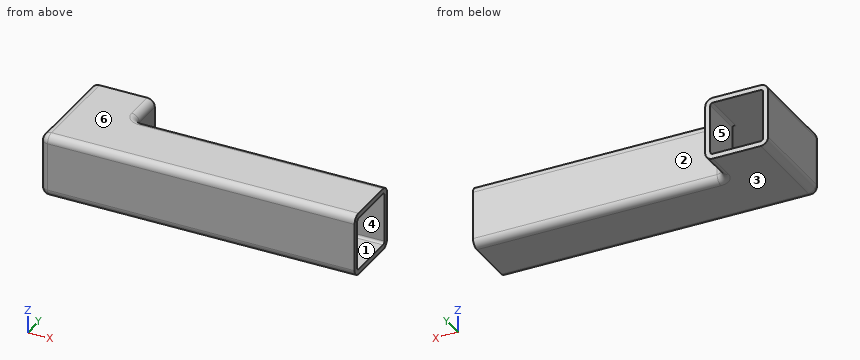
from build123d import *

# Parameters (mm, degrees)
SKETCH1_W           = 125
SKETCH1_H           = 40
BOSS_EXTRUDE1_DEPTH = 25
SKETCH2_W           = 100
SKETCH2_H           = 15
CUT_EXTRUDE1_DEPTH  = 25
SKETCH3_W           = 21
SKETCH3_H           = 21
CUT_EXTRUDE2_DEPTH  = 123
SKETCH4_W           = 21
SKETCH4_H           = 21
CUT_EXTRUDE3_DEPTH  = 38
FILLET3_R           = 1
FILLET4_R           = 1
FILLET5_R           = 1
FILLET6_R           = 1
FILLET7_R           = 1
FILLET8_R           = 1
FILLET9_R           = 3
FILLET11_R          = 3
FILLET12_R          = 3


with BuildPart() as part:
    # Sketch1 → Boss-Extrude1 (new body)
    with BuildSketch(Plane.XY):
        with Locations((62.5, 20)):
            Rectangle(SKETCH1_W, SKETCH1_H)
    extrude(amount=BOSS_EXTRUDE1_DEPTH)

    # Sketch2 → Cut-Extrude1 (cut)
    with BuildSketch(Plane.XY.offset(25)):
        with Locations((75, 32.5)):
            Rectangle(SKETCH2_W, SKETCH2_H)
    extrude(amount=-CUT_EXTRUDE1_DEPTH, mode=Mode.SUBTRACT)

    # Sketch3 → Cut-Extrude2 (cut)
    with BuildSketch(Plane(origin=(125, 0, 0), x_dir=(0, 0, -1), z_dir=(1, 0, 0))):
        with Locations((-12.5, 12.5)):
            Rectangle(SKETCH3_W, SKETCH3_H)
    extrude(amount=-CUT_EXTRUDE2_DEPTH, mode=Mode.SUBTRACT)

    # Sketch4 → Cut-Extrude3 (cut)
    with BuildSketch(Plane(origin=(0, 40, 0), x_dir=(1, 0, 0), z_dir=(0, 1, 0))):
        with Locations((12.5, -12.5)):
            Rectangle(SKETCH4_W, SKETCH4_H)
    extrude(amount=-CUT_EXTRUDE3_DEPTH, mode=Mode.SUBTRACT)

    # Fillet3
    fillet3_edges = [part.edges().sort_by_distance(p)[0] for p in [
        (2, 21, 2),
        (63.5, 2, 2),
    ]]
    fillet(fillet3_edges, radius=FILLET3_R)

    # Fillet4
    fillet4_edges = [part.edges().sort_by_distance(p)[0] for p in [
        (2, 21, 23),
        (63.5, 2, 23),
    ]]
    fillet(fillet4_edges, radius=FILLET4_R)

    # Fillet5
    fillet5_edges = [part.edges().sort_by_distance(p)[0] for p in [
        (74, 23, 2),
    ]]
    fillet(fillet5_edges, radius=FILLET5_R)

    # Fillet6
    fillet6_edges = [part.edges().sort_by_distance(p)[0] for p in [
        (74, 23, 23),
    ]]
    fillet(fillet6_edges, radius=FILLET6_R)

    # Fillet7
    fillet7_edges = [part.edges().sort_by_distance(p)[0] for p in [
        (23, 31, 23),
    ]]
    fillet(fillet7_edges, radius=FILLET7_R)

    # Fillet8
    fillet8_edges = [part.edges().sort_by_distance(p)[0] for p in [
        (23, 31, 2),
    ]]
    fillet(fillet8_edges, radius=FILLET8_R)

    # Fillet9
    fillet9_edges = [part.edges().sort_by_distance(p)[0] for p in [
        (25, 25, 12.5),
        (25, 32.5, 25),
        (75, 25, 25),
        (0, 20, 25),
        (62.5, 0, 25),
    ]]
    fillet(fillet9_edges, radius=FILLET9_R)

    # Fillet11
    fillet11_edges = [part.edges().sort_by_distance(p)[0] for p in [
        (76.5, 25, 0),
        (25.878679656, 25.878679656, 0),
        (25, 34, 0),
        (62.5, 0, 0),
        (0, 20, 0),
    ]]
    fillet(fillet11_edges, radius=FILLET11_R)

    # Fillet12
    # the kernel refuses this fillet: 3 mm, written as the material it takes off along each edge
    with BuildSketch(Plane(origin=(3, 3, 22), x_dir=(-1, 0, 0), z_dir=(0, -1, 0))) as fillet12_piece_1_section:
        Polygon((0, 0), (FILLET12_R, 0), (FILLET12_R, -FILLET12_R), (0, -FILLET12_R), align=None)
    fillet12_piece_1 = extrude(amount=FILLET12_R, mode=Mode.PRIVATE)
    fillet12_piece_1 = fillet12_piece_1 - Plane(origin=(3, 3, 22), x_dir=(0.7071067811865475, 0, -0.7071067811865475), z_dir=(0, -1, 0)) * Sphere(FILLET12_R, mode=Mode.PRIVATE)
    add(fillet12_piece_1, mode=Mode.SUBTRACT)
    with BuildSketch(Plane(origin=(3, 3, 3), x_dir=(-1, 0, 0), z_dir=(0, -1, 0))) as fillet12_piece_2_section:
        Polygon((0, 0), (FILLET12_R, 0), (FILLET12_R, FILLET12_R), (0, FILLET12_R), align=None)
    fillet12_piece_2 = extrude(amount=FILLET12_R, mode=Mode.PRIVATE)
    fillet12_piece_2 = fillet12_piece_2 - Plane(origin=(3, 3, 3), x_dir=(0.7071067811865475, 0, 0.7071067811865475), z_dir=(0, -1, 0)) * Sphere(FILLET12_R, mode=Mode.PRIVATE)
    add(fillet12_piece_2, mode=Mode.SUBTRACT)
    with BuildSketch(Plane(origin=(0, 0, 3), x_dir=(1, 0, 0), z_dir=(0, 0, 1))) as fillet12_piece_3:
        with BuildLine():
            CenterArc((FILLET12_R, FILLET12_R), FILLET12_R, 180, 90)
            Line((0, FILLET12_R), (0, 0))
            Line((0, 0), (FILLET12_R, 0))
        make_face()
    extrude(amount=19, mode=Mode.SUBTRACT)


solid = part.part
Can you work these out from the model? Positions are in its coordinate system, mm. Face numbers are marked on the shaded views. A direction names the side the tool comes from. Give positions to 0.01 mm unless a question says otherwise; leave off trailing zeros. Order: outer loops, then holes, each group sorted by start corner. A loop starts at its lowest first (then second) coordinate and runs counter-clockwise, first axis right, second up. Notation, with made-up numbers: M 43.25,-18.75 L 60.25,-18.75 A20 cw 60.25,-6.75 Z; hole C 56.5,-21.5 d2. An arc over 180 degrees is marked long. Use a Markdown table: item, result. Add a question column.
Item 1: For the marked faces 5 and 6, which set-ups out of +Z, -Z, +X, -X, +Y, -Y let a thin tool reach every point of the face, with its end or its side?
Item 2: Will these pins go through, and if not, where does the flat tip stop? pin 1 (3.5 mm diameter, centred on y = 34, z = 12.5, fed in from +X); pin 2 (3 mm diameter, centred on x = 28, y = 29, fed in from -Z); pin 3 (15 mm diameter, centred on x = 81, z = 16, fed in from +Y); pin 4 (10 mm diameter, centred on x = 29.5, y = 28, fed in from +Z).
Item 3: We'd pull the mould along Y, two halves only. Please class the marked faces 1, 2, 3 and 4: +Y half, -Y half, draft (parallel to the pull), parting line (faces both ways), or undercut.
Item 4: Suppose I cut it at A-A (z = 20.5). List the corners of the cut face in (x, y) for me.
Item 5: Suppose I cut it at B-B (x = 84). List the corners of the cut face in (y, z) for me.
Item 6: Suppose I cut it at C-C (y = 16). List the corners of the cut face in (x, z) for me.
Item 7: If I drill on L1, parallel to Z at x = 108, y = 12.5, over which ranges is the centre line in solid material (lowest first)? Write a range as [from, to].
Answer sheet:
| question | item | result |
|---|---|---|
| 1 | face 5 | +Y |
| 1 | face 6 | +Z, +X, -X, +Y, -Y |
| 2 | pin 1 | stops at x = 25 |
| 2 | pin 2 | passes through |
| 2 | pin 3 | stops at y = 25 |
| 2 | pin 4 | stops at z = 24.83 |
| 3 | face 1 | undercut |
| 3 | face 2 | +Y half |
| 3 | face 3 | draft |
| 3 | face 4 | undercut |
| 4 | outline | M 0,3 A3 ccw 3,0 L 125,0 L 125,2 L 2,2 L 2,40 L 0,40 Z; M 23,23 L 125,23 L 125,25 L 28,25 A3 cw 25,28 L 25,40 L 23,40 Z |
| 5 | outline | M 0,3 A3 ccw 3,0 L 22,0 A3 ccw 25,3 L 25,22 A3 ccw 22,25 L 3,25 A3 ccw 0,22 Z; hole M 2,3 A1 ccw 3,2 L 22,2 A1 ccw 23,3 L 23,22 A1 ccw 22,23 L 3,23 A1 ccw 2,22 Z |
| 6 | outline | M 0,3 A3 ccw 3,0 L 125,0 L 125,2 L 3,2 A1 cw 2,3 L 2,22 A1 cw 3,23 L 125,23 L 125,25 L 3,25 A3 ccw 0,22 Z |
| 7 | L1 | z = [0, 2], [23, 25] |
